Answer from the drawing. Dimensions are ordinates in mm from the lowest x, y and z of the part. A direction names the side the tool comes from. Coordinates: 2 decimals unless noted, no trailing zeros. Loops run counter-clockwise (first coordinate to the right, second up) from the corner with the lowest first, then second, coordinate; pieces in that order, holes last.
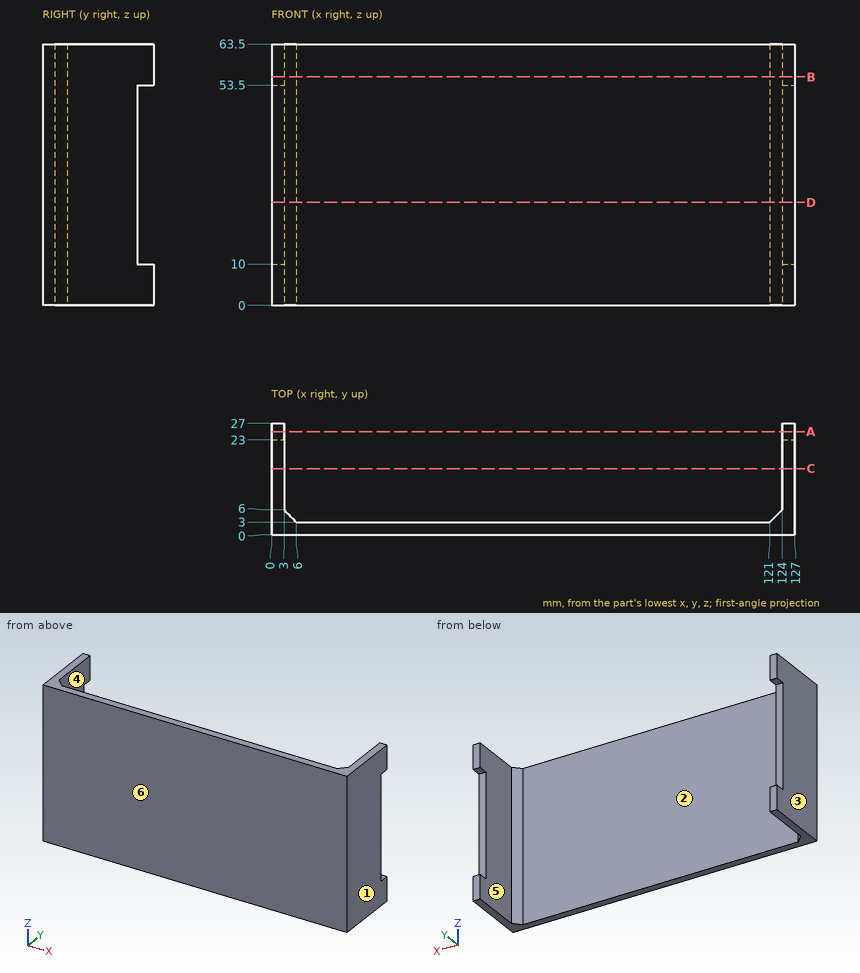
Item 1: A cutting plane is placed at C-C on y = 16. Determine the outline of the cut face in (x, z).
Numbers:
outline: (0, 0) - (3, 0) - (3, 63.5) - (0, 63.5) - close; (124, 0) - (127, 0) - (127, 63.5) - (124, 63.5) - close
Item 2: A cutting plane is placed at A-A on y = 25. Determine the outline of the cut face in (x, z), then the cut area to 3 significant figures.
Numbers:
outline: (0, 0) - (3, 0) - (3, 10) - (0, 10) - close; (0, 53.5) - (3, 53.5) - (3, 63.5) - (0, 63.5) - close; (124, 0) - (127, 0) - (127, 10) - (124, 10) - close; (124, 53.5) - (127, 53.5) - (127, 63.5) - (124, 63.5) - close
area: 120 mm2
Item 3: Find the intervals of material crossed by line 1 along X through (y, z) = (10, 52.5); line 2 along Y through (x, z) = (13, 60.5); line 3 along X through (y, z) = (3.5, 37), in increasing order.
Numbers:
line 1: x = 0 to 3, 124 to 127
line 2: y = 0 to 3
line 3: x = 0 to 5.5, 121.5 to 127
Item 4: Given pin 1 (1.5 mm diameter, centred on x = 103.5, z = 41.5, fed in from +Y); pin 2 (3.5 mm diameter, centred on x = 1.5, z = 36, fed in from +Y), each flat-ended and moving along its own axis, determine where each tip first touches the part or whether it passes through.
Numbers:
pin 1: stops at y = 3
pin 2: stops at y = 23
Item 5: Determine the mould class of the marked faces 1, 2, 3 and 4 for opening direction X: released by +X, released by -X, zero draft, split by the parting line, or undercut.
Numbers:
face 1: released by +X
face 2: undercut
face 3: released by -X
face 4: undercut
Item 6: A cutting plane is placed at B-B on z = 55.5. Determine the outline of the cut face in (x, y).
Numbers:
outline: (0, 0) - (127, 0) - (127, 27) - (124, 27) - (124, 6) - (121, 3) - (6, 3) - (3, 6) - (3, 27) - (0, 27) - close
Item 7: A cutting plane is placed at D-D on z = 25. Determine the outline of the cut face in (x, y).
Numbers:
outline: (0, 0) - (127, 0) - (127, 23) - (124, 23) - (124, 6) - (121, 3) - (6, 3) - (3, 6) - (3, 23) - (0, 23) - close
Item 8: Which of the six approach directions +Z, -Z, +X, -X, +Y, -Y give full straight-line access (tool end or side, diameter ignored) to the marked faces 5 and 6?
Numbers:
face 5: +Z, -Z, +Y
face 6: +Z, -Z, +X, -X, -Y
